Design review of the part built by this model. Coordinates are the model's own, in mm. A direction names the side the tool comes from. Give positions to 0.01 mm unless a question says otherwise; leave off trailing zeros. Write each loop counter-clockwise with the first axis right and the second up, starting at its lowest first coordinate (ties: lowest second). Pieces come first, ordered by that corner, then holes. Notation, with made-up numbers: (-15, 33) -> (13, 33) arc R24 cw to (13, 70) -> close; hole circle Ø7 at (75.5, 78). An arc over 180 degrees is marked (long way). Use CSV: the item, a comma, the result in double quotes.
```python
from build123d import *

# Parameters (mm, degrees)
SKETCH1_W           = 30
SKETCH1_H           = 60
BOSS_EXTRUDE1_DEPTH = 7
SKETCH2_W           = 30
SKETCH2_H           = 7
BOSS_EXTRUDE2_DEPTH = 35
BOSS_EXTRUDE3_DEPTH = 3
SKETCH4_W           = 30
SKETCH4_H           = 7
BOSS_EXTRUDE4_DEPTH = 33
SKETCH5_R           = 11
SKETCH5_R_2         = 7
BOSS_EXTRUDE5_DEPTH = 12
CUT_EXTRUDE1_START  = -12
SKETCH6_R           = 7
CUT_EXTRUDE1_DEPTH  = 12


with BuildPart() as part:
    # Sketch1 → Boss-Extrude1 (new body)
    with BuildSketch(Plane.XY):
        Rectangle(SKETCH1_W, SKETCH1_H)
    extrude(amount=BOSS_EXTRUDE1_DEPTH)

    # Sketch2 → Boss-Extrude2 (add)
    with BuildSketch(Plane.XY.offset(7)):
        with Locations((0, -26.5)):
            Rectangle(SKETCH2_W, SKETCH2_H)
    extrude(amount=BOSS_EXTRUDE2_DEPTH)

    # Sketch3 → Boss-Extrude3 (add, symmetric)
    with BuildSketch(Plane(origin=(0, 0, 0), x_dir=(0, 0, -1), z_dir=(1, 0, 0))):
        Polygon((-7, -23), (-7, 19), (-30, -23), align=None)
    extrude(amount=BOSS_EXTRUDE3_DEPTH, both=True)

    # Sketch4 → Boss-Extrude4 (add)
    with BuildSketch(Plane(origin=(0, 0, 0), x_dir=(-1, 0, 0), z_dir=(0, 0, -1))):
        with Locations((0, 26.5)):
            Rectangle(SKETCH4_W, SKETCH4_H)
    extrude(amount=BOSS_EXTRUDE4_DEPTH)

    # Sketch5 → Boss-Extrude5 (add)
    with BuildSketch(Plane(origin=(0, 30, 0), x_dir=(1, 0, 0), z_dir=(0, 1, 0))):
        with Locations(Location((0, 13, 0), (0, 0, 90))):
            Circle(SKETCH5_R)
        with Locations(Location((0, 13, 0), (0, 0, 270))):
            Circle(SKETCH5_R_2, mode=Mode.SUBTRACT)
    extrude(amount=BOSS_EXTRUDE5_DEPTH)

    # Sketch6 → Cut-Extrude1 (cut)
    with BuildSketch(Plane(origin=(0, 30, 0), x_dir=(1, 0, 0), z_dir=(0, 1, 0)).offset(CUT_EXTRUDE1_START)):
        with Locations(Location((0, 13, 0), (0, 0, 270))):
            Circle(SKETCH6_R)
    extrude(amount=CUT_EXTRUDE1_DEPTH, mode=Mode.SUBTRACT)


solid = part.part
```
(1) For line 1 along Z through (x, y) = (0, 28); line 2 along X through (y, z) = (31, -13); line 3 along X through (y, z) = (9, 9.5), list the stretches that pass through material, from the lowest coordinate up. Write a range as [from, to].
Established:
line 1,"z = [-33, -20], [-6, 7]"
line 2,"x = [-11, -7], [7, 11]"
line 3,"x = [-3, 3]"
(2) Take a section at B-B (z = -13). Write out the cut boundary in (x, y), then the cut area to 3 significant figures.
Established:
outline,"(-15, 23) -> (-7, 23) -> (-7, 42) -> (-11, 42) -> (-11, 30) -> (-15, 30) -> close; (7, 23) -> (15, 23) -> (15, 30) -> (11, 30) -> (11, 42) -> (7, 42) -> close"
area,"208 mm2"
(3) Clearance check with flat-ended pins moving along their axes: pin 1 (9 mm diameter, centred on x = 4.5, z = -19.5, fed in from -Y); pin 2 (1 mm diameter, centred on x = 1, y = -12, fed in from +Z); pin 3 (12 mm diameter, centred on x = 5, y = 16.5, fed in from -Z). State where each tip first meets the part, or that it passes through.
Established:
pin 1,"stops at y = 23"
pin 2,"stops at z = 24.25"
pin 3,"stops at z = 0"
(4) Mouldability with a two-part tool opening along Z and no side actions: class faces 5 (the face through (0, -26, 42)), 6 (the face through (0, 32, -20)), 7 (the face through (-3, -11, 14)), 8 (the face through (0, -3, 0)) as +Z half, -Z half, draft (parallel to the pull), parting line (faces both ways), or undercut.
Established:
face 5,"+Z half"
face 6,"undercut"
face 7,"draft"
face 8,"-Z half"
(5) Tool access review of faces 1 (the face through (3, -11, 14)), 2 (the face through (-4, 4, 7)), 3 (the face through (10.74, 35.92, -10.62)), 4 (the face through (4, 23, -20)): name each direction out of +Z, -Z, +X, -X, +Y, -Y from which nothing blocks a thin tool from reaching the whole face with its end or side.
Established:
face 1,"+Z, +X, +Y"
face 2,"+Z, +Y"
face 3,"+Y"
face 4,"-Z, +X, -X, -Y"
(6) Take a section at C-C (y = 28). Write out the cut boundary in (x, z), then the cut area to 3 significant figures.
Established:
outline,"(-15, -33) -> (15, -33) -> (15, 7) -> (-15, 7) -> close; hole circle Ø14 at (0, -13)"
area,"1,050 mm2"
(7) Take a section at D-D (y = 8.5). Write out the cut boundary in (x, z), then the cut area to 4 significant figures.
Established:
outline,"(-15, 0) -> (15, 0) -> (15, 7) -> (3, 7) -> (3, 12.75) -> (-3, 12.75) -> (-3, 7) -> (-15, 7) -> close"
area,"244.5 mm2"
(8) Take a section at A-A (x = 0). Write out the cut boundary in (y, z).
Established:
outline,"(-30, 0) -> (23, 0) -> (23, -6) -> (42, -6) -> (42, -2) -> (30, -2) -> (30, 7) -> (19, 7) -> (-23, 30) -> (-23, 42) -> (-30, 42) -> close; (23, -33) -> (30, -33) -> (30, -24) -> (42, -24) -> (42, -20) -> (23, -20) -> close"
